Read the model definition and answer for the solid it produces. Units are mm, in the model's axes. Face numbers are marked on the shaded views. A direction names the side the tool comes from. Coordinates: 2 decimals unless noted, no trailing zeros. Loops run counter-clockwise (first coordinate to the right, second up) from the corner with the lowest first, then second, coordinate; pieces in that order, holes last. Notation, with made-up numbers: (-37, -17) - (10, -17) arc R8 cw to (10, -7) - close; hole circle Ø3 at (-8.5, 70). An arc over 180 degrees is marked (long way). Use one line per item in the form item = value. Start each with the question number.
1) A cutting plane is placed at A-A (z = 9.5). Give the vertices of the cut face in (x, y).
2) A cutting plane is placed at B-B (z = 0.75). Give the vertices of the cut face in (x, y).
3) Consider line 1 (Y direction, x = 0, z = 9.8); line 2 (Z direction, x = -6.25, y = 4.5); line 3 (X direction, y = 5.5, z = 1.75). Determine where each line is inside the solid, lowest interval first.
4) Which of the six approach directions +Z, -Z, +X, -X, +Y, -Y give full straight-line access (tool end or side, diameter ignored) to the marked faces 4 and 5?
5) A cutting plane is placed at C-C (z = 6.5). Give the vertices of the cut face in (x, y).
6) The mould has two halves that part along Y. Classify the marked faces 1, 2 and 3: released by +Y, released by -Y, zero draft, split by the parting line, or undercut.
7) Each of these flat-tipped pins is pushed along its axis until it touches: P1, Ø6, axis at x = 7.5, y = 8, coming from the +Z side; P2, Ø6.5, axis at x = 0, y = 0, coming from the -Z side; P3, Ø4, axis at y = -2, z = 7, coming from the +X side; P4, Ø3, axis at x = 7, y = -8.5, coming from the +Z side. Where does it stop, or does it pass through?
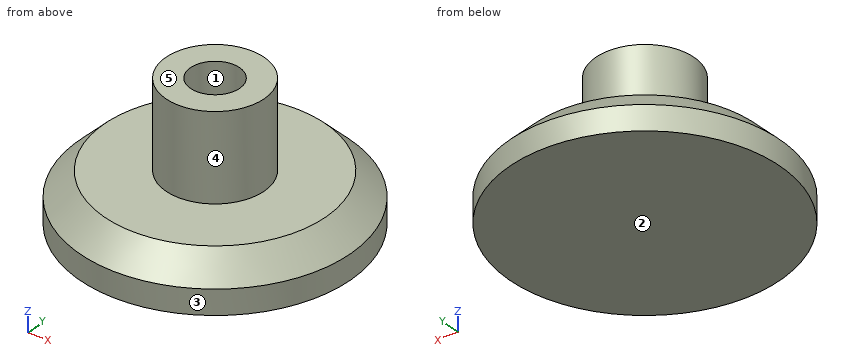
from build123d import *

# Parameters (mm, degrees)
F0_R     = 11
F1_DEPTH = 4
F2_SIZE  = 2
F3_R     = 4
F4_DEPTH = 7
F6_D     = 4
F6_DEPTH = 4
F6_TIP   = 1.2017212381


with BuildPart() as f1:
    # F0 (on Top) → F1 (new body)
    with BuildSketch(Plane.XY):
        Circle(F0_R)
    extrude(amount=F1_DEPTH)

    # F2
    f2_edges = [f1.edges().sort_by_distance(p)[0] for p in [
        (-11, 0, 4),
    ]]
    chamfer(f2_edges, length=F2_SIZE)

    # F3 (on face) → F4 (join)
    with BuildSketch(Plane.XY.offset(4)):
        Circle(F3_R)
    extrude(amount=F4_DEPTH)

    # F6
    with Locations(Plane.XY.offset(11)):
        with Locations((0, 0)):
            Hole(F6_D / 2, depth=F6_DEPTH)
            with Locations((0, 0, -(F6_DEPTH + F6_TIP / 2))):  # 118° drill point
                Cone(0, F6_D / 2, F6_TIP, mode=Mode.SUBTRACT)


solid = f1.part
Found:
q1.outline = circle Ø8 at (0, 0); hole circle Ø4 at (0, 0)
q2.outline = circle Ø22 at (0, 0)
q3.line_1 = -4 to -2, 2 to 4
q3.line_2 = 0 to 4
q3.line_3 = -9.53 to 9.53
q4.face_4 = +Z
q4.face_5 = +Z, +X, -X, +Y, -Y
q5.outline = circle Ø8 at (0, 0); hole circle Ø2.34 at (0, 0)
q6.face_1 = undercut
q6.face_2 = zero draft
q6.face_3 = split by the parting line
q7.P1 = 4
q7.P2 = 0
q7.P3 = 4
q7.P4 = 3.49
